from build123d import *

# Parameters (mm, degrees)
F0_W        = 909.2783331871
F0_H        = 769.7594761848
F0_R        = 87.1640503321
F1_DEPTH    = 509.82533
F2_W        = 512.1824108064
F2_H        = 509.82533
F3_DEPTH    = 167.38894
F4_T1_DEPTH = 509.82533


# Not quite as in the source:
# - a fillet or chamfer that OpenCascade refuses, or shapes differently, is made with other operations: its cross-section is extruded or revolved along the edge and cut away or added


with BuildPart() as f1:
    # F0 (on Top) → F1 (new body)
    with BuildSketch(Plane.XY):
        with Locations((-191.2371218204, -78.1787037849)):
            Rectangle(F0_W, F0_H)
        with Locations((-441.408932209, 54.1237108409)):
            Circle(F0_R, mode=Mode.SUBTRACT)
    extrude(amount=F1_DEPTH)

    # F2 (on face) → F3 (cut)
    with BuildSketch(Plane.YZ.offset(263.4020447731)):
        with Locations((-206.9672364742, 254.912665)):
            Rectangle(F2_W, F2_H)
    extrude(amount=-F3_DEPTH, mode=Mode.SUBTRACT)

    # F4: fillet of radius 192.8795849713 on 1 edges, made by hand

    # F4_s2 → F4_t1 (join)
    with BuildSketch(Plane.XY):
        with BuildLine():
            ThreePointArc((263.4020447731, 49.1239689291), (143.7734985232, -15.0088679899), (96.0131047731, -142.0637956315))
            Line((96.0131047731, -142.0637956315), (96.0131047731, 49.1239689291))
            Line((96.0131047731, 49.1239689291), (263.4020447731, 49.1239689291))
        make_face()
    extrude(amount=F4_T1_DEPTH)


solid = f1.part
The listing builds one solid part. Answer for the finished solid, in the listing's coordinates (mm). A direction names the side the tool comes from. Round coordinates to 2 decimals unless told otherwise and drop trailing zeros. Loops run counter-clockwise (first coordinate to the right, second up) from the corner with the lowest first, then second, coordinate; pieces in that order, holes last. Notation, with made-up numbers: M 41.5,15 L 50.5,15 A20 ccw 50.5,52 Z; hole C 70.5,13 d10. An arc over 180 degrees is marked long. Write each question's results on one line, items separated by ' | '. Start each with the question number.
1) Find section D-D on y = -20. Write down the section's boundary in (x, z).
2) Find section A-A on y = 87. Write down the section's boundary in (x, z).
3) Find section C-C on y = -358.5. Write down the section's boundary in (x, z).
4) Find section B-B on z = 463.5. Write down the section's boundary in (x, y).
5) Straight lines are drawn through the part: probe 1 along X at (y, z) = (-333.5, 179.5); probe 2 along Y at (x, z) = (-431, 316.5); probe 3 along X at (y, z) = (116.5, 326). For each, find the intervals that lie inside material, in ascending order.
6) Determine the mould class of faces 3 (the cylindrical face through (145.06, -13.554, 251.344)), 4 (the flat face through (-185, -73, 509.825)), 5 (the flat face through (-645.876, -84, 251)), 6 (the cylindrical face through (-528.49, 57.96, 251.34)) for opening direction X: pulls with the +X half, pulls with the -X half, needs draft (parallel to the pull), parting line crosses it, or undercut.
7) This flat-tipped pin is pushed along its axis until it touches: pin 1 (12 mm diameter, centred on y = 21, z = 145, fed in from +X). Where does it stop, or does it pass through?
8) Which of the six approach directions +Z, -Z, +X, -X, +Y, -Y give full straight-line access (tool end or side, diameter ignored) to faces 1 (the flat face through (96.013, -305, 258)), 2 (the flat face through (-280, -463.058, 251))?
Final values:
1) outline: M -645.88,0 L -487.27,0 L -487.27,509.83 L -645.88,509.83 Z; M -395.55,0 L 139.55,0 L 139.55,509.83 L -395.55,509.83 Z
2) outline: M -645.88,0 L -522.14,0 L -522.14,509.83 L -645.88,509.83 Z; M -360.68,0 L 263.4,0 L 263.4,509.83 L -360.68,509.83 Z
3) outline: M -645.88,0 L 96.01,0 L 96.01,509.83 L -645.88,509.83 Z
4) outline: M -645.88,-463.06 L 96.01,-463.06 L 96.01,-142.06 A192.88 cw 263.4,49.12 L 263.4,306.7 L -645.88,306.7 Z; hole C -441.41,54.12 d174.33
5) probe 1: -645.88 to 96.01 | probe 2: -463.06 to -32.42, 140.66 to 306.7 | probe 3: -645.88 to -502.29, -380.53 to 263.4
6) face 3: pulls with the +X half | face 4: needs draft | face 5: pulls with the -X half | face 6: undercut
7) pin 1: x = 196.05
8) face 1: +Z, -Z, +X, -Y | face 2: +Z, -Z, +X, -X, -Y
